The drawing under review shows one solid part. Ordinate dimensions are in mm from its lowest x, y, z. Give positions to 0.01 mm unless a question says otherwise; leave off trailing zeros. Loops run counter-clockwise (first coordinate to the right, second up) from the corner with the lowest first, then second, coordinate; pieces in that order, holes last. Notation, with made-up numbers: (32, -27) - (55, -27) arc R26 ccw to (55, -5) - close; hole circle Ø8 at (10.5, 58). An arc over 180 degrees is marked (long way). One line per item, written item: value. Start each with the question number.
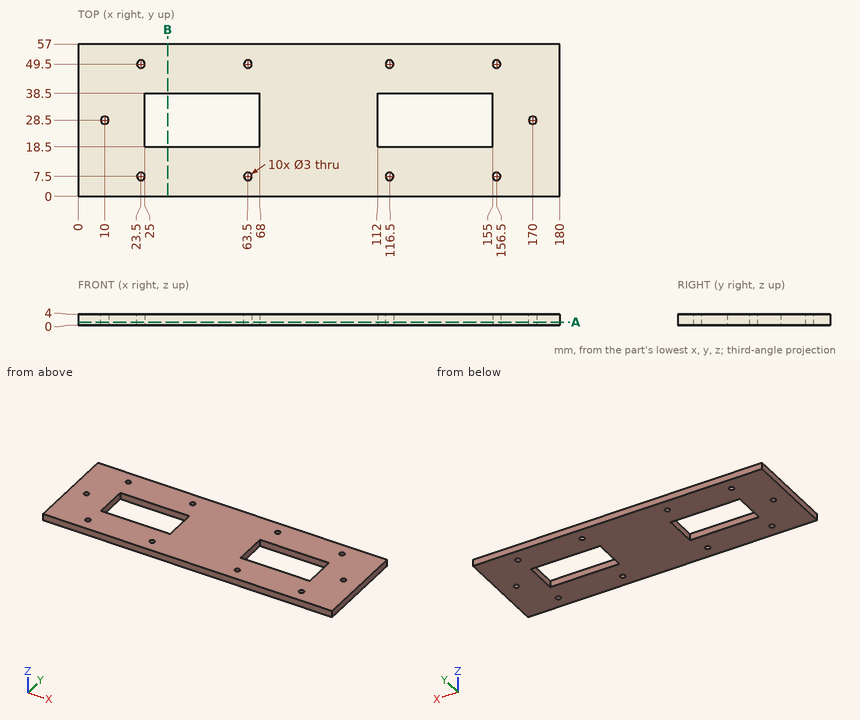
(1) Take a section at B-B on x = 33.5. State the section outline as (y, z) points, and give its area (3 significant figures).
(2) For pin 1 Ø2.5 at (x, y) = (63.5, 49.5) entering from +Z, flat-tipped, find the tip position at first contact; note if it passes through.
(3) Take a section at A-A on z = 1.1. State how many separate pieces and enclosed holes the cut face has, and give its area (3 significant figures).
(4) To check wall thickness, follow L1, parallel to Y at x = 116.5, z = 2.4; L2, parallel to X at y = 38, z = 0.7; L3, parallel to Y at x = 170, z = 0.8. State the ranges of each line that lie inside material, in increasing order. Write a range as from..to.
Here are the results:
1. outline: (0, 0) - (18.5, 0) - (18.5, 4) - (0, 4) - close; (38.5, 0) - (57, 0) - (57, 4) - (38.5, 4) - close
1. area: 148 mm²
2. pin 1: through
3. separate pieces: 1
3. enclosed holes: 12
3. area: 8,470 mm²
4. L1: 0..6, 9..18.5, 38.5..48, 51..57
4. L2: 0..25, 68..112, 155..180
4. L3: 0..27, 30..57
